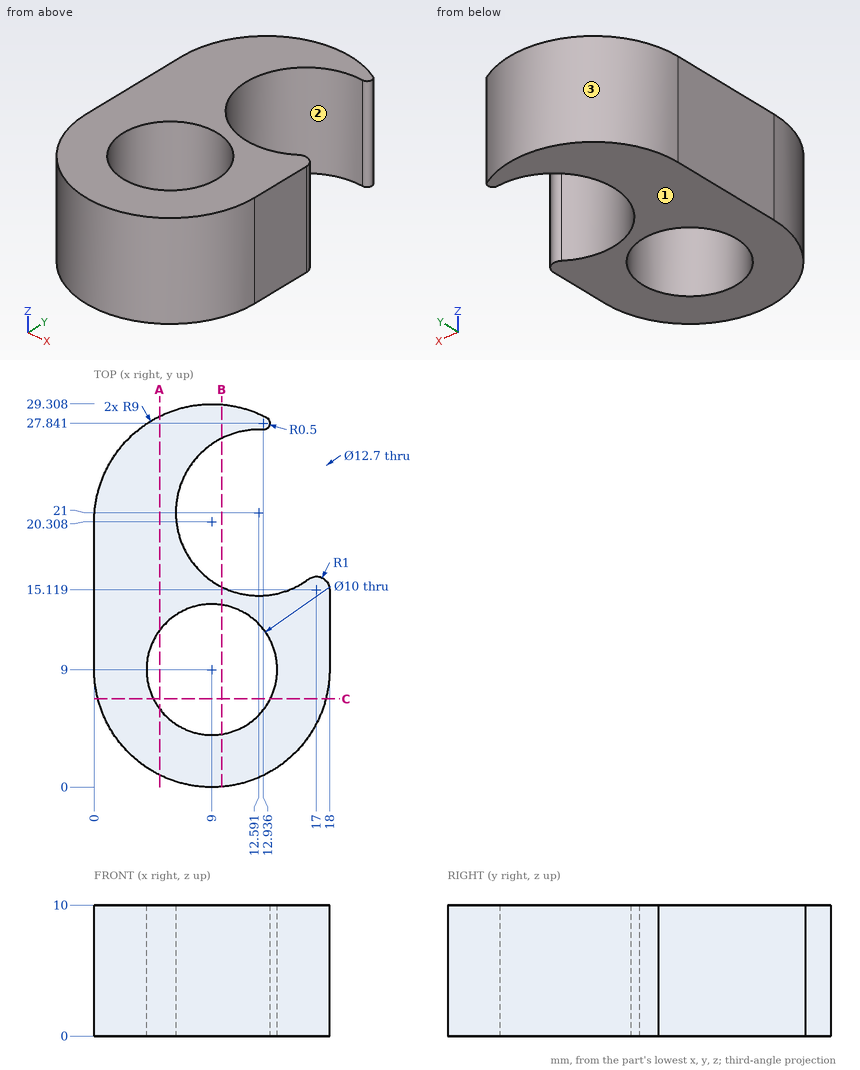
Print and shaded views of the part. All mm, measured from the part's lowest x, y and z. Round coordinates to 2 decimals unless told otherwise and drop trailing zeros. Write each loop counter-clockwise with the first axis right and the second up, starting at its lowest first coordinate (ties: lowest second). Pieces come first, ordered by that corner, then holes. Notation, with made-up numbers: (-7, 16) -> (1, 16) arc R5 ccw to (1, 22) -> close; hole circle Ø5 at (76, 46.25). An arc over 180 degrees is marked (long way). Answer in a Markdown table with one row per item. Add a question column.
Item 1: Drill centre lines: line 1 (Y direction, x = 9, z = 8.25); line 2 (Y direction, x = 9.5, z = 6) (1 decimal); line 3 (X direction, y = 7.75, z = 2). Where is each one in solid material? Low to high. Write a range as from..to.
Item 2: Mould opens along Y. For the marked faces 1, 2 and 3 say: pulls with the +Y half, pulls with the -Y half, needs draft (parallel to the pull), parting line crosses it, or undercut.
Item 3: Saw through at A-A, the plane x = 5. Write the cut outline in (y, z), then the cut area to 3 significant figures.
Item 4: Drop a flat-ended pin along its axis: pin 1 Ø3 at (y, z) = (15, 3) entering from -X. Give the stop position or say it passes through.
Item 5: Saw through at B-B, the plane x = 9.75. Write the cut outline in (y, z).
Item 6: Saw through at C-C, the plane y = 6.75. Write the cut outline in (x, z) (1 decimal).
Findings below:
| question | item | result |
|---|---|---|
| 1 | line 1 | y = 0..4, 14..15.76, 26.24..29.31 |
| 1 | line 2 | y = 0..4, 14..15.5, 26.5..29.3 |
| 1 | line 3 | x = 0.09..4.16, 13.84..17.91 |
| 2 | face 1 | needs draft |
| 2 | face 2 | undercut |
| 2 | face 3 | pulls with the +Y half |
| 3 | outline | (0.94, 0) -> (6, 0) -> (6, 10) -> (0.94, 10) -> close; (12, 0) -> (28.37, 0) -> (28.37, 10) -> (12, 10) -> close |
| 3 | area | 214 mm^2 |
| 4 | pin 1 | stops at x = 0 |
| 5 | outline | (0.03, 0) -> (4.06, 0) -> (4.06, 10) -> (0.03, 10) -> close; (13.94, 0) -> (15.32, 0) -> (15.32, 10) -> (13.94, 10) -> close; (26.68, 0) -> (29.28, 0) -> (29.28, 10) -> (26.68, 10) -> close |
| 6 | outline | (0.3, 0) -> (4.5, 0) -> (4.5, 10) -> (0.3, 10) -> close; (13.5, 0) -> (17.7, 0) -> (17.7, 10) -> (13.5, 10) -> close |
